Verification items for the finished model (mm, model axes). A direction names the side the tool comes from. Round coordinates to 2 decimals unless told otherwise and drop trailing zeros. Order: outer loops, then holes, each group sorted by start corner. A loop starts at its lowest first (then second) coordinate and runs counter-clockwise, first axis right, second up. Notation, with made-up numbers: (81.25, 30.25) -> (123.25, 30.25) arc R29 cw to (123.25, 65.25) -> close; hole circle Ø2 at (47, -12.75). An arc over 180 degrees is marked (long way). Put each result on its own line as item: value.
from build123d import *

# Parameters (mm, degrees)
F1_DEPTH = 25
F2_R     = 5
F3_R     = 5
F4_R     = 4.99999


# Not quite as in the source:
# - a fillet or chamfer is up to 0.001 mm smaller than in the source, because OpenCascade refuses the exact size


with BuildPart() as f1:
    # F0 (on Front) → F1 (new body)
    with BuildSketch(Plane.XZ):
        Polygon((-125, 35), (-125, 45), (-165, 45), (-165, -45), (-125, -45), (-125, -35), (-155, -35), (-155, 35), align=None)
        Polygon((125, -75), (125, 75), (-125, 75), (-125, 45), (-125, 35), (-125, -35), (-125, -45), (-125, -75), align=None)
    extrude(amount=F1_DEPTH)

    # F2
    f2_edges = [f1.edges().sort_by_distance(p)[0] for p in [
        (-125, -12.5, 45),
        (-165, -12.5, 45),
        (-165, -12.5, -45),
        (-125, -12.5, -45),
        (-125, -12.5, -35),
        (-155, -12.5, -35),
        (-155, -12.5, 35),
        (-125, -12.5, 35),
        (-125, -12.5, 75),
        (-125, -12.5, -75),
        (125, -12.5, -75),
        (125, -12.5, 75),
    ]]
    fillet(f2_edges, radius=F2_R)

    # F3
    f3_edges = [f1.edges().sort_by_distance(p)[0] for p in [
        (-145, -25, 45),
    ]]
    fillet(f3_edges, radius=F3_R)

    # F4 (radius 5 in the source; OpenCascade refuses exactly that, so slightly less here)
    f4_edges = [f1.edges().sort_by_distance(p)[0] for p in [
        (-140, -25, 35),
        (-145, 0, -45),
        (-140, 0, -35),
    ]]
    fillet(f4_edges, radius=F4_R)


solid = f1.part
Item 1: Tool access check on faces 1 (the cylindrical face through (-123, -1, 0)), 2 (the cylindrical face through (-154, -13, 33)), 3 (the cylindrical face through (-140, -24, -37)). Record the directions out of +Z, -Z, +X, -X, +Y, -Y that give a thin tool (end or side, any length) a straight path to the whole face; none if there is none.
Check sheet entries:
face 1: +Y
face 2: +Y, -Y
face 3: -Y
Item 2: Material ranges on L1, parallel to Z at x = -147.5, y = -12.5; L2, parallel to X at y = -7.75, z = 5; L3, parallel to X at y = -21.75, z = 22.5, recorded low to high. Write a range as [from, to].
Check sheet entries:
L1: z = [-45, -35], [35, 45]
L2: x = [-165, -155], [-125, 125]
L3: x = [-164.68, -155.32], [-124.68, 124.68]
Item 3: Release check for a two-part mould opening along Z. For faces 4 (the cylindrical face through (2, -23, -74)), 5 (the cylindrical face through (-157, -1, 0)), 6 (the cylindrical face through (-123, -1, -60)) record: +Z half, -Z half, draft (parallel to the pull), parting line (faces both ways), or undercut.
Check sheet entries:
face 4: -Z half
face 5: undercut
face 6: draft
Item 4: Gauge pin test, flat ends, axial feed: pin 1 Ø4.5 at (y, z) = (-11, -59.5) entering from -X; pin 2 Ø4.5 at (x, y) = (-151.5, -12) entering from +Z; pin 3 Ø12 at (x, y) = (-139, -15) entering from -Z. Record the tip position at first contact, or that the pin passes through.
Check sheet entries:
pin 1: stops at x = -125
pin 2: stops at z = 45
pin 3: stops at z = -45
Item 5: Section check C-C on y = -11. Record the boundary of the cut face in (x, z).
Check sheet entries:
outline: (-165, -40) arc R5 ccw to (-160, -45) -> (-130, -45) arc R5 cw to (-125, -50) -> (-125, -70) arc R5 ccw to (-120, -75) -> (120, -75) arc R5 ccw to (125, -70) -> (125, 70) arc R5 ccw to (120, 75) -> (-120, 75) arc R5 ccw to (-125, 70) -> (-125, 50) arc R5 cw to (-130, 45) -> (-160, 45) arc R5 ccw to (-165, 40) -> close; hole (-155, -30) arc R5 ccw to (-150, -35) -> (-130, -35) arc R5 ccw to (-125, -30) -> (-125, 30) arc R5 ccw to (-130, 35) -> (-150, 35) arc R5 ccw to (-155, 30) -> close
